Could you check a few things on this model? Use its own coordinates, in mm. Face numbers are marked on the shaded views. A direction names the side the tool comes from. Give positions to 0.01 mm unless a question says otherwise; leave off trailing zeros. Write each loop counter-clockwise with the first axis right and the second up, starting at its lowest first coordinate (ties: lowest second). Pieces come first, ordered by that corner, then holes. Notation, with made-up numbers: M 88.25,-21.5 L 98.25,-21.5 A13 cw 98.25,-16.5 Z; hole C 1,52.5 d9. An arc over 180 degrees is marked long. One line per item, written item: value.
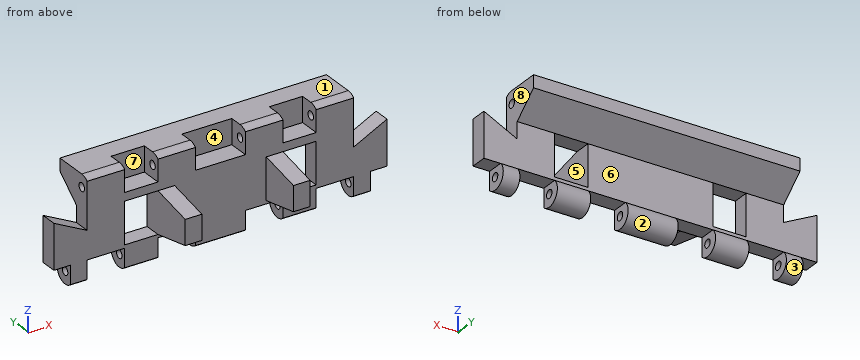
```python
from build123d import *

# Parameters (mm, degrees)
SALIENTE_EXTRUIR1_DEPTH      = 1
SALIENTE_EXTRUIR1_DEPTH_BACK = 1
CROQUIS2_R                   = 0.5
SALIENTE_EXTRUIR2_DEPTH      = 40
CORTAR_EXTRUIR1_DEPTH        = 40
CROQUIS6_R                   = 0.5
CORTAR_EXTRUIR2_DEPTH        = 2
CROQUIS7_R                   = 0.5
CORTAR_EXTRUIR3_DEPTH        = 2
CROQUIS9_R                   = 0.5
SALIENTE_EXTRUIR3_DEPTH      = 32
CORTAR_EXTRUIR4_DEPTH        = 36
CROQUIS11_W                  = 4.5
CROQUIS11_H                  = 2.236067978
CROQUIS11_H_2                = 0.381966011
CORTAR_EXTRUIR5_DEPTH        = 36
CROQUIS14_W                  = 4
CROQUIS14_H                  = 1.5
CROQUIS14_H_2                = 1
CROQUIS14_W_2                = 6
CORTAR_EXTRUIR6_DEPTH        = 3
SALIENTE_EXTRUIR4_DEPTH      = 2
SALIENTE_EXTRUIR5_DEPTH      = 2


with BuildPart() as part:
    # Croquis1 → Saliente-Extruir1 (new body, two sides)
    with BuildSketch(Plane(origin=(0, 0, 0), x_dir=(1, 0, 0), z_dir=(0, 1, 0))) as saliente_extruir1_sk:
        Polygon((-16, 0), (-20, 0), (-20, -5), (-16, -3), align=None)
        Polygon((-11.5, 0), (-16, 0), (-16, -3), (-16, -6), (16, -6), (16, -3), (16, 0), (11.5, 0), (11.5, -5), (7.5, -5), (7.5, 0), (-7.5, 0), (-7.5, -5), (-11.5, -5), align=None)
        Polygon((16, 0), (16, -3), (20, -5), (20, 0), align=None)
    extrude(amount=SALIENTE_EXTRUIR1_DEPTH)
    extrude(saliente_extruir1_sk.sketch, amount=-SALIENTE_EXTRUIR1_DEPTH_BACK)

    # Croquis2 → Saliente-Extruir2 (add)
    with BuildSketch(Plane(origin=(20, 0, 0), x_dir=(0, 0, -1), z_dir=(1, 0, 0))):
        with BuildLine():
            Line((0, -1), (0.381966011, -1))
            ThreePointArc((0.381966011, -1), (3, 0), (0.381966011, 1))
            Line((0.381966011, 1), (0, 1))
            Line((0, 1), (0, 0))
            Line((0, 0), (0, -1))
        make_face()
        with Locations((1.5, 0)):
            Circle(CROQUIS2_R, mode=Mode.SUBTRACT)
    extrude(amount=-SALIENTE_EXTRUIR2_DEPTH)

    # Croquis5 → Cortar-Extruir1 (cut)
    with BuildSketch(Plane(origin=(20, 0, 0), x_dir=(0, 0, -1), z_dir=(1, 0, 0))):
        with BuildLine():
            Line((2.618033989, -1), (0.381966011, -1))
            ThreePointArc((0.381966011, -1), (1.5, -1.5), (2.618033989, -1))
        make_face()
    extrude(amount=-CORTAR_EXTRUIR1_DEPTH, mode=Mode.SUBTRACT)

    # Croquis6 → Cortar-Extruir2 (cut)
    with BuildSketch(Plane(origin=(20, 0, 0), x_dir=(0, 0, -1), z_dir=(1, 0, 0))):
        with BuildLine():
            ThreePointArc((2.618033989, -1), (2.5, 1.118033989), (0.381966011, 1))
            Line((0.381966011, 1), (0.381966011, -1))
            Line((0.381966011, -1), (2.618033989, -1))
        make_face()
        with Locations((1.5, 0)):
            Circle(CROQUIS6_R, mode=Mode.SUBTRACT)
    extrude(amount=-CORTAR_EXTRUIR2_DEPTH, mode=Mode.SUBTRACT)

    # Croquis7 → Cortar-Extruir3 (cut)
    with BuildSketch(Plane.ZY.offset(20)):
        with BuildLine():
            Line((-0.381966011, -1), (-0.381966011, 1))
            ThreePointArc((-0.381966011, 1), (-2.5, 1.118033989), (-2.618033989, -1))
            Line((-2.618033989, -1), (-0.381966011, -1))
        make_face()
        with Locations((-1.5, 0)):
            Circle(CROQUIS7_R, mode=Mode.SUBTRACT)
    extrude(amount=-CORTAR_EXTRUIR3_DEPTH, mode=Mode.SUBTRACT)

    # Croquis9 → Saliente-Extruir3 (add)
    with BuildSketch(Plane.ZY.offset(16)):
        with BuildLine():
            Line((6, 0), (6, -1))
            Line((6, -1), (6.381966011, -1))
            ThreePointArc((6.381966011, -1), (8.035233135, -1.401258538), (9, 0))
            Line((9, 0), (9, 4))
            Line((9, 4), (7.5, 4))
            Line((7.5, 4), (5, 1))
            Line((5, 1), (6, 1))
            Line((6, 1), (6, 0))
        make_face()
        with Locations((7.5, 0)):
            Circle(CROQUIS9_R, mode=Mode.SUBTRACT)
    extrude(amount=-SALIENTE_EXTRUIR3_DEPTH)

    # Croquis10 → Cortar-Extruir4 (cut)
    with BuildSketch(Plane.ZY.offset(16)):
        with BuildLine():
            Line((8.618033989, -1), (6.381966011, -1))
            ThreePointArc((6.381966011, -1), (7.5, -1.5), (8.618033989, -1))
        make_face()
    extrude(amount=-CORTAR_EXTRUIR4_DEPTH, mode=Mode.SUBTRACT)

    # Croquis11 → Cortar-Extruir5 (cut)
    with BuildSketch(Plane.XZ.offset(1)):
        with Locations((13.75, -1.5)):
            Rectangle(CROQUIS11_W, CROQUIS11_H)
        with Locations((5.25, -1.5)):
            Rectangle(CROQUIS11_W, CROQUIS11_H)
        with Locations((-5.25, -1.5)):
            Rectangle(CROQUIS11_W, CROQUIS11_H)
        with Locations((-13.75, -1.5)):
            Rectangle(CROQUIS11_W, CROQUIS11_H)
        with Locations((-13.75, -2.809016995)):
            Rectangle(CROQUIS11_W, CROQUIS11_H_2)
        with Locations((-5.25, -2.809016995)):
            Rectangle(CROQUIS11_W, CROQUIS11_H_2)
        with Locations((5.25, -2.809016995)):
            Rectangle(CROQUIS11_W, CROQUIS11_H_2)
        with Locations((13.75, -2.809016995)):
            Rectangle(CROQUIS11_W, CROQUIS11_H_2)
    extrude(amount=-CORTAR_EXTRUIR5_DEPTH, mode=Mode.SUBTRACT)

    # Croquis14 → Cortar-Extruir6 (cut)
    with BuildSketch(Plane.XY.offset(9)):
        with Locations((-9.5, 0.75)):
            Rectangle(CROQUIS14_W, CROQUIS14_H)
        with Locations((-9.5, -0.5)):
            Rectangle(CROQUIS14_W, CROQUIS14_H_2)
        with Locations((0, 0.75)):
            Rectangle(CROQUIS14_W_2, CROQUIS14_H)
        with Locations((0, -0.5)):
            Rectangle(CROQUIS14_W_2, CROQUIS14_H_2)
        with Locations((9.5, 0.75)):
            Rectangle(CROQUIS14_W, CROQUIS14_H)
        with Locations((9.5, -0.5)):
            Rectangle(CROQUIS14_W, CROQUIS14_H_2)
    extrude(amount=-CORTAR_EXTRUIR6_DEPTH, mode=Mode.SUBTRACT)

    # Croquis15 → Saliente-Extruir4 (add)
    with BuildSketch(Plane.ZY.offset(7.5)):
        Polygon((5, -1), (0, -1), (1, -6), (4, -6), align=None)
    extrude(amount=-SALIENTE_EXTRUIR4_DEPTH)

    # Croquis16 → Saliente-Extruir5 (add)
    with BuildSketch(Plane(origin=(7.5, 0, 0), x_dir=(0, 0, -1), z_dir=(1, 0, 0))):
        Polygon((0, -1), (-5, -1), (-4, -6), (-1, -6), align=None)
    extrude(amount=-SALIENTE_EXTRUIR5_DEPTH)


solid = part.part
```
1) Please list where these lines run through material, in increasing order: L1, parallel to X at y = -4.5, z = 2.75; L2, parallel to Y at x = -1.65, z = -1.5; L3, parallel to Y at x = 4, z = 4.5. Write a range as from..to.
Outcome:
L1: x = -7.5..-5.5, 5.5..7.5
L2: y = -1..-0.5, 0.5..1.5
L3: y = -1..1
2) We'd pull the mould along Z, two halves only. Please class the marked faces 1, 2, 3 and 4: pulls with the +Z half, pulls with the -Z half, needs draft (parallel to the pull), parting line crosses it, or undercut.
Outcome:
face 1: pulls with the +Z half
face 2: undercut
face 3: parting line crosses it
face 4: needs draft
3) On a 3-axis mill with a long thin cutter (end or side, diameter ignored), from which of +Z, -Z, +X, -X, +Y, -Y can I reach the whole of each face in a straight line? I mean the marked faces 5, 6, 7 and 8. Say none if no direction works.
Outcome:
face 5: +Y, -Y
face 6: +X, -X, +Y
face 7: +Z, -Y
face 8: +Z, +Y, -Y
4) If we section it at C-C, the plane z = 3.5: Write out the boundary of the cut face in (x, y).
Outcome:
outline: M -20,-1 L -17,-1 L -17,1 L -20,1 Z; M -16,-1 L -11.5,-1 L -11.5,1 L -16,1 Z; M -7.5,-6 L -5.5,-6 L -5.5,-1 L 5.5,-1 L 5.5,-6 L 7.5,-6 L 7.5,1 L -7.5,1 Z; M 11.5,-1 L 16,-1 L 16,1 L 11.5,1 Z; M 17,-1 L 20,-1 L 20,1 L 17,1 Z
5) I'm going to push flat-ended pins straight in: pin 1 (1 mm diameter, centred on y = -4.5, z = 3.5, fed in from +X); pin 2 (3 mm diameter, centred on y = 0.5, z = -2, fed in from -X); pin 3 (2.5 mm diameter, centred on y = -3.5, z = 3, fed in from -X); pin 4 (1.5 mm diameter, centred on x = 0, y = -2, fed in from +Z). Where does each tip first touch, or does it pass through?
Outcome:
pin 1: stops at x = 7.5
pin 2: stops at x = -18
pin 3: stops at x = -7.5
pin 4: passes through
6) If we section it at B-B, the plane y = -3.5: Write out the boundary of the cut face in (x, z).
Outcome:
outline: M -7.5,0.5 L -5.5,0.5 L -5.5,4.5 L -7.5,4.5 Z; M 5.5,0.5 L 7.5,0.5 L 7.5,4.5 L 5.5,4.5 Z
7) If we section it at A-A, the plane x = 11: Write out the boundary of the cut face in (y, z), then the cut area to 3 significant figures.
Outcome:
outline: M -1,-2.62 A1.5 ccw 1,-0.38 L 1,0 L -1,0 Z; M -1,5 L 1,5 L 4,7.5 L 4,9 L 1.5,9 L 1.5,6 L -1,6 Z; hole C 0,-1.5 d1
area: 14.5 mm^2
8) If we section it at D-D, the plane x = 0.5: Write out the boundary of the cut face in (y, z).
Outcome:
outline: M -1,-2.62 A1.5 ccw 1,-0.38 L 1,5 L 4,7.5 L 4,9 L 1.5,9 L 1.5,6 L -1,6 Z; hole C 0,-1.5 d1
